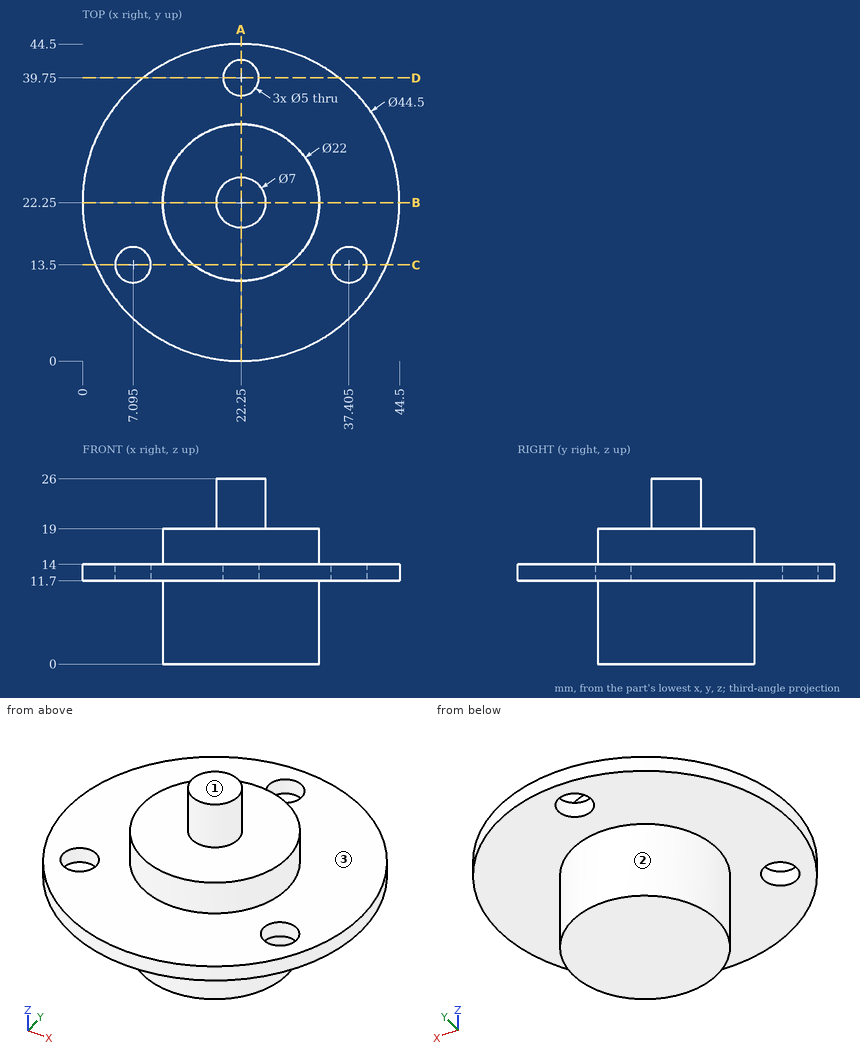
Geometry: see drawing. Coordinates: mm, zero at the bounding-box minimum. A direction names the side the tool comes from. Give positions to 0.01 mm unless a question says otherwise; leave off trailing zeros. Loops run counter-clockwise (first coordinate to the right, second up) from the corner with the lowest first, then second, coordinate; pieces in that order, holes last. Notation, with made-up numbers: M 49.5,78.25 L 100.5,78.25 A22 ccw 100.5,89.25 Z; hole C 19,25.5 d5. An arc over 180 degrees is marked long. Use one line per item in the form item = value.
1. Section query A-A, the plane x = 22.25. Return the cut outline in (y, z).
Numbers:
outline = M 0,11.7 L 11.25,11.7 L 11.25,0 L 33.25,0 L 33.25,11.7 L 37.25,11.7 L 37.25,14 L 33.25,14 L 33.25,19 L 25.75,19 L 25.75,26 L 18.75,26 L 18.75,19 L 11.25,19 L 11.25,14 L 0,14 Z; M 42.25,11.7 L 44.5,11.7 L 44.5,14 L 42.25,14 Z
2. Section query D-D, the plane y = 39.75. Return the cut outline in (x, z).
Numbers:
outline = M 8.51,11.7 L 19.75,11.7 L 19.75,14 L 8.51,14 Z; M 24.75,11.7 L 35.99,11.7 L 35.99,14 L 24.75,14 Z
3. Section query B-B, the plane y = 22.25. Return the cut outline in (x, z).
Numbers:
outline = M 0,11.7 L 11.25,11.7 L 11.25,0 L 33.25,0 L 33.25,11.7 L 44.5,11.7 L 44.5,14 L 33.25,14 L 33.25,19 L 25.75,19 L 25.75,26 L 18.75,26 L 18.75,19 L 11.25,19 L 11.25,14 L 0,14 Z
4. Reachability of the marked faces 1, 2 and 3 from +Z, -Z, +X, -X, +Y, -Y: full face, straight path, thin tool, end or side. Return the list, or none.
Numbers:
face_1 = +Z, +X, -X, +Y, -Y
face_2 = -Z
face_3 = +Z
5. Line query: L1, parallel to Y at x = 22.25, z = 13.4; L2, parallel to Z at x = 2, y = 20; L3, parallel to Z at x = 27, y = 14. Output: solid intervals per line, ascending.
Numbers:
L1 = 0 to 37.25, 42.25 to 44.5
L2 = 11.7 to 14
L3 = 0 to 19
6. Section query C-C, the plane y = 13.5. Return the cut outline in (x, z) (1 decimal).
Numbers:
outline = M 1.8,11.7 L 4.6,11.7 L 4.6,14 L 1.8,14 Z; M 9.6,11.7 L 15.6,11.7 L 15.6,0 L 28.9,0 L 28.9,11.7 L 34.9,11.7 L 34.9,14 L 28.9,14 L 28.9,19 L 15.6,19 L 15.6,14 L 9.6,14 Z; M 39.9,11.7 L 42.7,11.7 L 42.7,14 L 39.9,14 Z
7. First-contact query: pin 1 (11 mm diameter, centred on x = 18.5, y = 25.5, fed in from +Z); pin 2 (8 mm diameter, centred on x = 23.5, y = 31.5, fed in from +Z); pin 3 (8 mm diameter, centred on y = 34.5, z = 15, fed in from -X); pin 4 (1.5 mm diameter, centred on x = 33.5, y = 16.5, fed in from +Z). Flat tips, straight axial feed; report the tip coordinate or a pass-through.
Numbers:
pin_1 = 26
pin_2 = 19
pin_3 = 1.64
pin_4 = 14
